from build123d import *

# Parameters (mm, degrees)
BOSS_EXTRUDE1_DEPTH  = 0.125
SKETCH4_W            = 5
SKETCH4_H            = 3
CUT_EXTRUDE2_DEPTH   = 186.440185774
LPATTERN3_COUNT      = 4
LPATTERN3_PITCH      = 11
LPATTERN3_COUNT_DIR2 = 2
LPATTERN3_PITCH_DIR2 = 173


with BuildPart() as part:
    # Sketch2 → Boss-Extrude1 (new, symmetric)
    with BuildSketch(Plane.XY):
        Polygon((0, 0), (5, 0), (173, 22), (178, 22), (178, 52), (0, 52), align=None)
    extrude(amount=BOSS_EXTRUDE1_DEPTH, both=True)

    # Sketch4 → Cut-Extrude2 (cut, through all)
    with BuildSketch(Plane.XY.offset(0.125)):
        with Locations((175.5, 42.5)):
            Rectangle(SKETCH4_W, SKETCH4_H)
    cut_extrude2 = extrude(amount=-CUT_EXTRUDE2_DEPTH, mode=Mode.SUBTRACT)

    # LPattern3: Cut-Extrude2 4 × 2
    with Locations(*[(-j * LPATTERN3_PITCH_DIR2, -i * LPATTERN3_PITCH, 0) for i in range(LPATTERN3_COUNT) for j in range(LPATTERN3_COUNT_DIR2) if (i, j) != (0, 0)]):
        add(cut_extrude2, mode=Mode.SUBTRACT)


solid = part.part
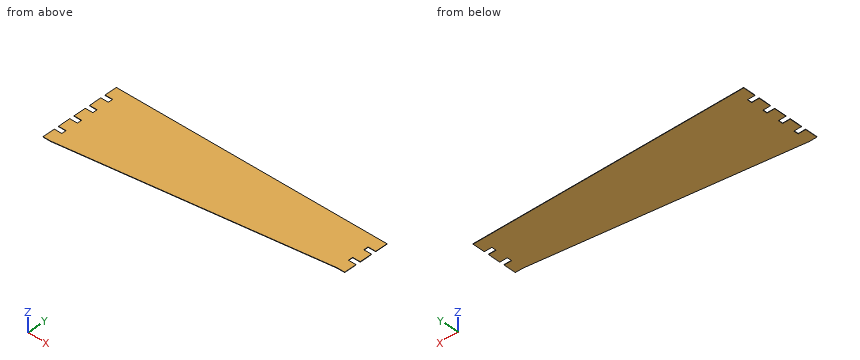
Source: CAD feature listing. Evaluate the final solid. Frame: model axes, mm. Coordinates: 2 decimals unless noted, no trailing zeros. Write each loop counter-clockwise with the first axis right and the second up, starting at its lowest first coordinate (ties: lowest second). Pieces come first, ordered by that corner, then holes. Notation, with made-up numbers: M 52.25,28.5 L 78.25,28.5 A24 cw 78.25,47.5 Z; hole C 44,30 d1. An arc over 180 degrees is marked long. Use a Markdown table: item, result.
1) Section B-B, the plane y = 5.5. Output: boundary loops of the cut face in (x, z) (3 decimals), then the cut area to 4 significant figures.
Conclusion:
| item | result |
|---|---|
| outline | M 0,-0.125 L 47,-0.125 L 47,0.125 L 0,0.125 Z |
| area | 11.75 mm^2 |
2) Ray query, L1, parallel to Y at x = 75, z = -0.05; L2, parallel to Y at x = 42.5, z = 0. Return the intervals inside material, ascending.
Conclusion:
| item | result |
|---|---|
| L1 | y = 9.17 to 52 |
| L2 | y = 4.91 to 52 |
3) Section C-C, the plane x = 117.5. Output: boundary loops of the cut face in (y, z) (3 decimals), then the cut area to 3 significant figures.
Conclusion:
| item | result |
|---|---|
| outline | M 14.732,-0.125 L 52,-0.125 L 52,0.125 L 14.732,0.125 Z |
| area | 9.32 mm^2 |
